CAD build for the part. Positions are in the model's coordinates, mm. Give positions to 0.01 mm unless a question says otherwise; leave off trailing zeros. Write each loop counter-clockwise with the first axis right and the second up, starting at its lowest first coordinate (ties: lowest second). Pieces come first, ordered by that corner, then holes. Notation, with made-up numbers: (18, -19) -> (65, -19) arc R23 cw to (65, 9) -> close; hole circle Ø5 at (70.25, 88). An arc over 180 degrees is marked (long way). Answer in a Markdown table with one row per item. Add a question column.
```python
from build123d import *

# Parameters (mm, degrees)
SKETCH1_R           = 2.54
SKETCH1_R_2         = 1.905
SKETCH1_R_3         = 6.35
BOSS_EXTRUDE1_DEPTH = 1.5875
FILLET1_R           = 5.08
FILLET2_R           = 2.54


with BuildPart() as part:
    # Sketch1 → Boss-Extrude1 (new body)
    with BuildSketch(Plane(origin=(0, 0, 0), x_dir=(1, 0, 0), z_dir=(0, 1, 0))):
        Polygon((69.85, 63.5), (4.445, 63.5), (4.445, 36.576), (-4.445, 36.576), (-4.445, 63.5), (-69.85, 63.5), (-69.85, -63.5), (69.85, -63.5), align=None)
        with Locations((-62.484, 56.134)):
            Circle(SKETCH1_R, mode=Mode.SUBTRACT)
        with Locations((-62.484, -56.134)):
            Circle(SKETCH1_R, mode=Mode.SUBTRACT)
        with Locations((62.484, 56.134)):
            Circle(SKETCH1_R, mode=Mode.SUBTRACT)
        with Locations((62.484, -56.134)):
            Circle(SKETCH1_R, mode=Mode.SUBTRACT)
        with Locations((50.8, -8.304005887)):
            Circle(SKETCH1_R_2, mode=Mode.SUBTRACT)
        with Locations((50.8, 32.589994113)):
            Circle(SKETCH1_R_2, mode=Mode.SUBTRACT)
        with Locations((50.8, 6.173994113)):
            Circle(SKETCH1_R_3, mode=Mode.SUBTRACT)
        with BuildLine():
            Line((-9.779, 43.434), (-9.779, 36.322))
            ThreePointArc((-9.779, 36.322), (-11.811, 34.29), (-13.843, 36.322))
            Line((-13.843, 36.322), (-13.843, 43.434))
            ThreePointArc((-13.843, 43.434), (-11.811, 45.466), (-9.779, 43.434))
        make_face(mode=Mode.SUBTRACT)
        with BuildLine():
            Line((-9.779, 9.398), (-9.779, 2.286))
            ThreePointArc((-9.779, 2.286), (-11.811, 0.254), (-13.843, 2.286))
            Line((-13.843, 2.286), (-13.843, 9.398))
            ThreePointArc((-13.843, 9.398), (-11.811, 11.43), (-9.779, 9.398))
        make_face(mode=Mode.SUBTRACT)
    extrude(amount=-BOSS_EXTRUDE1_DEPTH)

    # Fillet1
    fillet1_edges = [part.edges().sort_by_distance(p)[0] for p in [
        (-69.85, -0.79375, -63.5),
        (69.85, -0.79375, -63.5),
        (69.85, -0.79375, 63.5),
        (-69.85, -0.79375, 63.5),
    ]]
    fillet(fillet1_edges, radius=FILLET1_R)

    # Fillet2
    fillet2_edges = [part.edges().sort_by_distance(p)[0] for p in [
        (-4.445, -0.79375, -63.5),
        (-4.445, -0.79375, -36.576),
        (4.445, -0.79375, -36.576),
        (4.445, -0.79375, -63.5),
    ]]
    fillet(fillet2_edges, radius=FILLET2_R)


solid = part.part
```
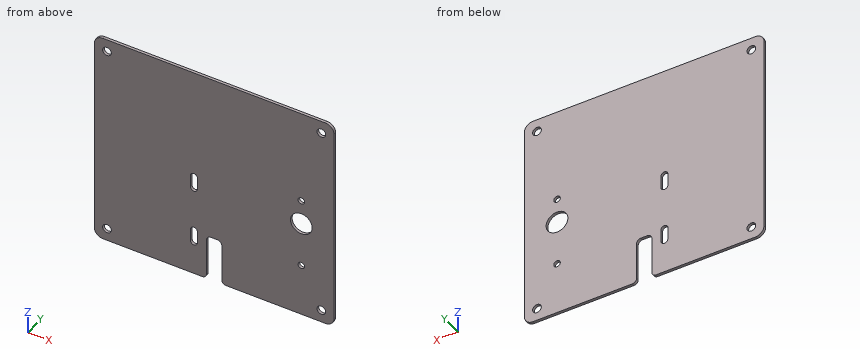
Item 1: Slice it at A-A, the plane x = 50.8. List the corners of the cut face in (y, z) (1 decimal), then the cut area to 3 significant figures.
Item 2: Drop a flat-ended pin along its axis: pin 1 Ø0.5 at (x, y) = (-0.5, -1) entering from -Z. Give the stop position or say it passes through.
Item 3: Slice it at B-B, the plane y = -1.2. State how many separate pieces and enclosed holes the cut face has, then the cut area to 3 significant figures.
Item 4: Probe L1, parallel to Z at x = -12, y = -0.85; L2, parallel to Z at x = 50.8, y = -1.2 (3 decimals); L3, parallel to X at y = -0.95, z = -37.5. List the from-to ranges inside material, lowest first. Write a range as from..to.
Answer key:
| question | item | result |
|---|---|---|
| 1 | outline | (-1.6, -63.5) -> (0, -63.5) -> (0, -34.5) -> (-1.6, -34.5) -> close; (-1.6, -30.7) -> (0, -30.7) -> (0, -12.5) -> (-1.6, -12.5) -> close; (-1.6, 0.2) -> (0, 0.2) -> (0, 6.4) -> (-1.6, 6.4) -> close; (-1.6, 10.2) -> (0, 10.2) -> (0, 63.5) -> (-1.6, 63.5) -> close |
| 1 | area | 169 mm² |
| 2 | pin 1 | stops at z = -36.58 |
| 3 | separate pieces | 1 |
| 3 | enclosed holes | 9 |
| 3 | area | 17,200 mm² |
| 4 | L1 | z = -63.5..-45.46, -34.3..-11.42, -0.26..63.5 |
| 4 | L2 | z = -63.5..-34.495, -30.685..-12.524, 0.176..6.399, 10.209..63.5 |
| 4 | L3 | x = -69.85..-13.84, -9.78..-3.86, 3.86..69.85 |
